from build123d import *

# Parameters (mm, degrees)
F0_R     = 139.7
F1_DEPTH = 431.8
F2_R     = 50.8
F3_SIZE2 = 121.0821650076
F3_SIZE  = 101.6
F4_R     = 101.6
F5_T     = -3.175


with BuildPart() as f1:
    # F0 (on Top) → F1 (new body)
    with BuildSketch(Plane.XY):
        Circle(F0_R)
    extrude(amount=F1_DEPTH)

    # F2
    f2_edges = [f1.edges().sort_by_distance(p)[0] for p in [
        (-139.7, 0, 0),
    ]]
    fillet(f2_edges, radius=F2_R)

    # F3
    f3_edges = [f1.edges().sort_by_distance(p)[0] for p in [
        (-139.7, 0, 431.8),
    ]]
    f3_side = f1.faces().sort_by_distance((0, 0, 431.8))[0]
    chamfer(f3_edges, length=F3_SIZE, length2=F3_SIZE2, reference=f3_side)

    # F4
    f4_edges = [f1.edges().sort_by_distance(p)[0] for p in [
        (-139.7, 0, 310.717835),
    ]]
    fillet(f4_edges, radius=F4_R)

    # F5
    f5_openings = [f1.faces().sort_by_distance(p)[0] for p in [
        (0, 0, 431.8),
    ]]
    offset(amount=F5_T, openings=f5_openings)


solid = f1.part
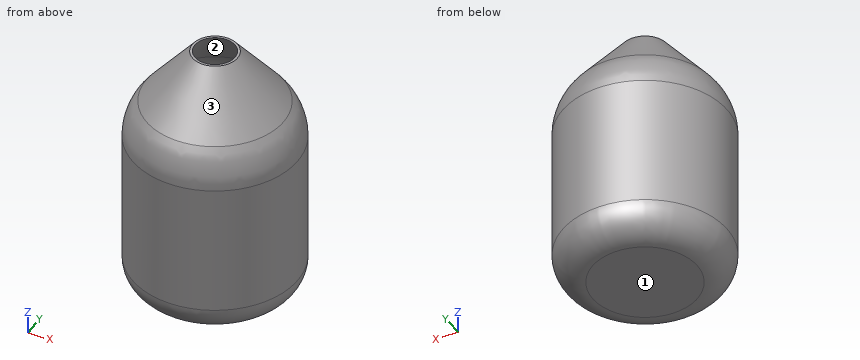
CAD build for the part. Positions are in the model's coordinates, mm. Face numbers are marked on the shaded views. Round coordinates to 2 decimals unless told otherwise and drop trailing zeros. Write each loop counter-clockwise with the first axis right and the second up, starting at its lowest first coordinate (ties: lowest second). Pieces come first, ordered by that corner, then holes. Notation, with made-up numbers: (74, 70.5) -> (132, 70.5) arc R24 ccw to (132, 94.5) -> close; hole circle Ø11 at (89, 10). An arc over 180 degrees is marked (long way). Answer as a JSON object with one key per item and string values.
(1) Pin check, flat tips, straight feed: P1, Ø8, axis at x = -95, y = 47.5, coming from the -Z side; P2, Ø10, axis at y = -34.5, z = 255, coming from the +X side; P3, Ø12, axis at y = -11, z = 176.5, coming from the +X side. Stop position of each tip, or through.
Reported:
{"P1": "stops at z = 1.78", "P2": "stops at x = 136.55", "P3": "stops at x = 139.61"}
(2) Two-plate mould, pull along Z, no slides. Class the marked faces 1, 2 and 3: +Z half, -Z half, draft (parallel to the pull), parting line (faces both ways), or undercut.
Reported:
{"face 1": "-Z half", "face 2": "undercut", "face 3": "+Z half"}
(3) Probe probe 1 along Y at (x, z) = (0, 197) (3 decimals); probe 2 along Z at (x, y) = (101, -5). List the from-to ranges inside material, lowest first. Write a range as [from, to].
Reported:
{"probe 1": "y = [-139.7, -136.525], [136.525, 139.7]", "probe 2": "z = [1.49, 4.77], [351.75, 356.69]"}
(4) Band-saw the part on A-A, the plane z = 108. List the corners of the cut face in (x, y) (3 decimals).
Reported:
{"outline": "circle Ø279.4 at (0, 0); hole circle Ø273.05 at (0, 0)"}
